from build123d import *

# Parameters (mm, degrees)
BOSS_EXTRUDE1_DEPTH = 20
SKETCH3_W           = 10
SKETCH3_H           = 20
BOSS_EXTRUDE2_DEPTH = 20
SKETCH4_R           = 2.5
CUT_EXTRUDE1_DEPTH  = 30


with BuildPart() as part:
    # Sketch2 → Boss-Extrude1 (new body)
    with BuildSketch(Plane(origin=(0, 0, 0), x_dir=(1, 0, 0), z_dir=(0, 1, 0))):
        Polygon((-190.55, 110.014093794), (190.55, 110.014093794), (0, -220.028187588), align=None)
    extrude(amount=BOSS_EXTRUDE1_DEPTH)

    # Sketch3 → Boss-Extrude2 (add)
    with BuildSketch(Plane(origin=(95.275, 0, 55.007046897), x_dir=(0.5, 0, -0.866025404), z_dir=(0.866025404, 0, 0.5))):
        with Locations((-10, 10)):
            Rectangle(SKETCH3_W, SKETCH3_H)
        with Locations((10, 10)):
            Rectangle(SKETCH3_W, SKETCH3_H)
    boss_extrude2 = extrude(amount=BOSS_EXTRUDE2_DEPTH)

    # Sketch4 → Cut-Extrude1 (cut)
    with BuildSketch(Plane(origin=(-7.5, 0, 12.990381057), x_dir=(0.866025404, 0, 0.5), z_dir=(-0.5, 0, 0.866025404))):
        with Locations((120.014093794, 10)):
            Circle(SKETCH4_R)
    cut_extrude1 = extrude(amount=-CUT_EXTRUDE1_DEPTH, mode=Mode.SUBTRACT)

    # Mirror1: Boss-Extrude2, Cut-Extrude1 across plane
    add(boss_extrude2.mirror(Plane(origin=(0, 0, 0), x_dir=(-0.866025404, 0, 0.5), z_dir=(0.5, 0, 0.866025404))))
    add(cut_extrude1.mirror(Plane(origin=(0, 0, 0), x_dir=(-0.866025404, 0, 0.5), z_dir=(0.5, 0, 0.866025404))), mode=Mode.SUBTRACT)

    # Mirror1 at the second plane: Boss-Extrude2, Cut-Extrude1 across plane
    add(boss_extrude2.mirror(Plane(origin=(0, 0, 0), x_dir=(0, 0, 1), z_dir=(1, 0, 0))))
    add(cut_extrude1.mirror(Plane(origin=(0, 0, 0), x_dir=(0, 0, 1), z_dir=(1, 0, 0))), mode=Mode.SUBTRACT)


solid = part.part
Verification items for the finished model (mm, model axes). A direction names the side the tool comes from. Coordinates: 2 decimals unless noted, no trailing zeros. Order: outer loops, then holes, each group sorted by start corner. A loop starts at its lowest first (then second) coordinate and runs counter-clockwise, first axis right, second up. Notation, with made-up numbers: M -26.75,70.25 L 12.25,70.25 A31 ccw 12.25,109.25 Z; hole C 65.5,10 d8. An arc over 180 degrees is marked long. Return JSON: item names as keys, results as strings.
1) Access from +Z, -Z, +X, -X, +Y, -Y to the whole of each face (thin tool, end or side, straight path). Record for faces 4 (the flat face through (-146.048, 9.86, -32.934)), 5 (the flat face through (15, 12, -122)), 6 (the flat face through (98.24, 12.08, 74.04)), 7 (the flat face through (5, 12, -122)), 8 (the flat face through (113.24, 12.08, 48.06)).
Answer list:
{"face 4": "-X, +Y, -Y", "face 5": "-Z, +X, +Y, -Y", "face 6": "+Z, +Y, -Y", "face 7": "-Z, +Y, -Y", "face 8": "+X, +Y, -Y"}
2) Gauge pin test, flat ends, axial feed: pin 1 (8 mm diameter, centred on y = 10, z = -120.01, fed in from -X); pin 2 (6 mm diameter, centred on y = 6, z = -117, fed in from +X); pin 3 (1.5 mm diameter, centred on y = 17, z = -94.5, fed in from +X); pin 4 (3 mm diameter, centred on y = 10, z = -120.01, fed in from +X). Record the tip position at first contact, or that the pin passes through.
Answer list:
{"pin 1": "x = -15", "pin 2": "x = 15", "pin 3": "x = 182.03", "pin 4": "through"}
3) Cross-section at A-A, the plane z = 110. Record the boundary of the cut face in (x, y).
Answer list:
{"outline": "M -63.52,0 L 63.52,0 L 63.52,20 L -63.52,20 Z"}
4) Cross-section at B-B, the plane x = -40. Record the boundary of the cut face in (y, z), and give its area (3 significant figures).
Answer list:
{"outline": "M 0,-110.01 L 20,-110.01 L 20,150.75 L 0,150.75 Z", "area": "5,220 mm2"}
5) Thickness scan on L1, parallel to X at y = 10.75, z = 53; L2, parallel to Z at x = 7, y = 10; L3, parallel to Z at x = 100, y = 17.25. Record the ranges inside material, lowest first. Write a range as [from, to].
Answer list:
{"L1": "[-119.53, -110.73], [-105.23, -101.8], [-96.43, 96.43], [101.8, 105.23], [110.73, 119.53]", "L2": "[-130.01, -122.51], [-117.51, 207.9]", "L3": "[-110.01, 51.96], [63.51, 75.06]"}
6) Release check for a two-part mould opening along X. For faces 1 (the flat face through (3, 20, 4)), 2 (the flat face through (-117.56, 10.14, 56.41)), 3 (the flat face through (104.4, 12.1, 54.5)) record: +X half, -X half, draft (parallel to the pull), parting line (faces both ways), or undercut.
Answer list:
{"face 1": "draft", "face 2": "-X half", "face 3": "undercut"}
